Can you work these out from the model? Positions are in its coordinate system, mm. A direction names the side the tool comes from. Round coordinates to 2 decimals unless told otherwise and drop trailing zeros. Order: outer loops, then holes, each group sorted by start corner. A loop starts at its lowest first (then second) coordinate and runs counter-clockwise, first axis right, second up. Notation, with made-up numbers: (78.25, 9.25) -> (103.25, 9.25) arc R28 cw to (103.25, 33.25) -> close; hole circle Ø5 at (70.25, 82). An arc over 180 degrees is marked (long way). One line per item, written item: value.
```python
from build123d import *

# Parameters (mm, degrees)
SKETCH1_W           = 38
SKETCH1_H           = 38
BOSS_EXTRUDE1_DEPTH = 2
SKETCH2_R           = 1.5
CUT_EXTRUDE1_DEPTH  = 27.944387171
BOSS_EXTRUDE2_DEPTH = 12.5
SKETCH4_R           = 9
CUT_EXTRUDE2_DEPTH  = 31.532769282
CUT_EXTRUDE3_START  = -2.5
CUT_EXTRUDE3_DEPTH  = 29.032769282
FILLET1_R           = 2


with BuildPart() as part:
    # Sketch1 → Boss-Extrude1 (new body)
    with BuildSketch(Plane(origin=(0, 0, 0), x_dir=(0, 1, 0), z_dir=(0, 0, 1))):
        Rectangle(SKETCH1_W, SKETCH1_H)
    extrude(amount=BOSS_EXTRUDE1_DEPTH)

    # Sketch2 → Cut-Extrude1 (cut, through all)
    with BuildSketch(Plane(origin=(0, 0, 0), x_dir=(1, 0, 0), z_dir=(0, 0, -1))):
        with Locations(Location((-16, 16, 0), (0, 0, 180))):
            Circle(SKETCH2_R)
        with Locations((-16, -16)):
            Circle(SKETCH2_R)
        with Locations((16, 16)):
            Circle(SKETCH2_R)
    extrude(amount=-CUT_EXTRUDE1_DEPTH, mode=Mode.SUBTRACT)

    # Sketch3 → Boss-Extrude2 (add)
    with BuildSketch(Plane.XY.offset(2)):
        with BuildLine():
            Line((-16, 9.5), (-16, -9.5))
            ThreePointArc((-16, -9.5), (-11.403805922, -11.403805922), (-9.5, -16))
            Line((-9.5, -16), (9.5, -16))
            ThreePointArc((9.5, -16), (11.403805922, -11.403805922), (16, -9.5))
            Line((16, -9.5), (16, 9.5))
            ThreePointArc((16, 9.5), (11.403805922, 11.403805922), (9.5, 16))
            Line((9.5, 16), (-9.5, 16))
            ThreePointArc((-9.5, 16), (-11.403805922, 11.403805922), (-16, 9.5))
        make_face()
    extrude(amount=BOSS_EXTRUDE2_DEPTH)

    # Sketch4 → Cut-Extrude2 (cut, through all)
    with BuildSketch(Plane.XY.offset(14.5)):
        Circle(SKETCH4_R)
    extrude(amount=-CUT_EXTRUDE2_DEPTH, mode=Mode.SUBTRACT)

    # Sketch5 → Cut-Extrude3 (cut, through all)
    with BuildSketch(Plane.XY.offset(14.5).offset(CUT_EXTRUDE3_START)):
        with BuildLine():
            Line((-13.5, -6.83484861), (-13.5, 6.83484861))
            ThreePointArc((-13.5, 6.83484861), (-9.282485579, 9.282485579), (-6.83484861, 13.5))
            Line((-6.83484861, 13.5), (6.83484861, 13.5))
            ThreePointArc((6.83484861, 13.5), (9.282485579, 9.282485579), (13.5, 6.83484861))
            Line((13.5, 6.83484861), (13.5, -6.83484861))
            ThreePointArc((13.5, -6.83484861), (9.282485579, -9.282485579), (6.83484861, -13.5))
            Line((6.83484861, -13.5), (-6.83484861, -13.5))
            ThreePointArc((-6.83484861, -13.5), (-9.282485579, -9.282485579), (-13.5, -6.83484861))
        make_face()
    extrude(amount=-CUT_EXTRUDE3_DEPTH, mode=Mode.SUBTRACT)

    # Fillet1
    fillet1_edges = [part.edges().sort_by_distance(p)[0] for p in [
        (-9.5, 16, 8.25),
        (-16, 9.5, 8.25),
        (-16, -9.5, 8.25),
        (-9.5, -16, 8.25),
        (9.5, -16, 8.25),
        (16, -9.5, 8.25),
        (16, 9.5, 8.25),
        (9.5, 16, 8.25),
    ]]
    fillet(fillet1_edges, radius=FILLET1_R)


solid = part.part
```
Q1. I want a section at B-B on y = 0. List the corners of the cut face in (x, z) for me, plus the area to 3 significant figures.
Answers below:
outline: (-19, 0) -> (-13.5, 0) -> (-13.5, 12) -> (-9, 12) -> (-9, 14.5) -> (-16, 14.5) -> (-16, 2) -> (-19, 2) -> close; (9, 12) -> (13.5, 12) -> (13.5, 0) -> (19, 0) -> (19, 2) -> (16, 2) -> (16, 14.5) -> (9, 14.5) -> close
area: 107 mm^2
Q2. On a 3-axis mill with a long thin cutter (end or side, diameter ignored), from which of +Z, -Z, +X, -X, +Y, -Y can I reach the whole of each face in a straight line? I mean faces 5 (the face through (-11.44, -11.37, 8.16)), 6 (the face through (-11.37, 11.44, 8.16)), 7 (the face through (0.2, 9.2, 12)), 8 (the face through (0, -16, 8)), 9 (the face through (11.37, -11.44, 8.16)). Say none if no direction works.
Answers below:
face 5: +Z, -X, -Y
face 6: +Z, -X, +Y
face 7: -Z
face 8: +Z, +X, -X, -Y
face 9: +Z, +X, -Y
Q3. Will these pins go through, and if not, where does the flat tip stop? pin 1 Ø2 at (x, y) = (4, 8) entering from -Z; pin 2 Ø3.5 at (y, z) = (2, 8.5) entering from -X; pin 3 Ø6 at (x, z) = (-2.5, 9.5) entering from +Y.
Answers below:
pin 1: z = 12
pin 2: x = -16
pin 3: y = 16
Q4. We'd pull the mould along X, two halves only. Please class faces 1 (the face through (0, -13.5, 6)), 2 (the face through (0, -19, 1)), 3 (the face through (-17.5, 15.93, 0.99)), 4 (the face through (19, 0, 1)): released by +X, released by -X, zero draft, split by the parting line, or undercut.
Answers below:
face 1: undercut
face 2: zero draft
face 3: undercut
face 4: released by +X
Q5. I want a section at D-D on x = -14. List the corners of the cut face in (y, z) for me, plus the area to 3 significant figures.
Answers below:
outline: (-19, 0) -> (19, 0) -> (19, 2) -> (9.82, 2) -> (9.82, 14.5) -> (-9.82, 14.5) -> (-9.82, 2) -> (-19, 2) -> close
area: 321 mm^2
Q6. I want a section at A-A on z = 3.5. List the corners of the cut face in (x, y) for me.
Answers below:
outline: (-16, -7.74) arc R2 ccw to (-14.47, -9.68) arc R6.5 cw to (-9.68, -14.47) arc R2 ccw to (-7.74, -16) -> (7.74, -16) arc R2 ccw to (9.68, -14.47) arc R6.5 cw to (14.47, -9.68) arc R2 ccw to (16, -7.74) -> (16, 7.74) arc R2 ccw to (14.47, 9.68) arc R6.5 cw to (9.68, 14.47) arc R2 ccw to (7.74, 16) -> (-7.74, 16) arc R2 ccw to (-9.68, 14.47) arc R6.5 cw to (-14.47, 9.68) arc R2 ccw to (-16, 7.74) -> close; hole (-13.5, -6.83) arc R9.5 cw to (-6.83, -13.5) -> (6.83, -13.5) arc R9.5 cw to (13.5, -6.83) -> (13.5, 6.83) arc R9.5 cw to (6.83, 13.5) -> (-6.83, 13.5) arc R9.5 cw to (-13.5, 6.83) -> close
Q7. Please list where these lines run through material, in increasing order: line 1 along Y through (x, z) = (-16, 1.45); line 2 along X through (y, z) = (-2.5, 9); line 3 along Y through (x, z) = (16, 1.25).
Answers below:
line 1: -19 to -17.5, -14.5 to 14.5, 17.5 to 19
line 2: -16 to -13.5, 13.5 to 16
line 3: -19 to -17.5, -14.5 to 19
